Here's how the part is built. I have some questions about the finished solid (model axes, mm). Give positions to 0.01 mm unless a question says otherwise; leave off trailing zeros. Order: outer loops, then holes, each group sorted by start corner. A loop starts at its lowest first (then second) coordinate and runs counter-clockwise, first axis right, second up.
from build123d import *

# Parameters (mm, degrees)
F0_R     = 75
F1_DEPTH = 8


with BuildPart() as f1:
    # F0 (on Top) → F1 (new body)
    with BuildSketch(Plane.XY):
        with BuildLine():
            ThreePointArc((-168.166967, -90.974196), (-117.487432, -76.990459), (-83, -37.309516))
            ThreePointArc((-83, -37.309516), (-48.512568, -76.990459), (2.166967, -90.974196))
            ThreePointArc((2.166967, -90.974196), (84.481738, -33.820644), (64.346717, 64.346717))
            ThreePointArc((64.346717, 64.346717), (-83, 125.379726), (-230.346717, 64.346717))
            ThreePointArc((-230.346717, 64.346717), (-250.481738, -33.820644), (-168.166967, -90.974196))
        make_face()
        with Locations((-166, 0)):
            Circle(F0_R, mode=Mode.SUBTRACT)
        with BuildLine():
            ThreePointArc((-75, 0), (0, 75), (75, 0))
            ThreePointArc((75, 0), (0, -75), (-75, 0))
        make_face(mode=Mode.SUBTRACT)
        with Locations((-166, 0)):
            Circle(F0_R)
        with BuildLine():
            ThreePointArc((2.166967, -90.974196), (-48.512568, -76.990459), (-83, -37.309516))
            ThreePointArc((-83, -37.309516), (-117.487432, -76.990459), (-168.166967, -90.974196))
            Line((-168.166967, -90.974196), (-83.238128, -92.997164))
            ThreePointArc((-83.238128, -92.997164), (-89.98637, -75.845236), (-73, -83))
            ThreePointArc((-73, -83), (-75.845236, -89.98637), (-82.761872, -92.997164))
            Line((-82.761872, -92.997164), (2.166967, -90.974196))
        make_face()
    extrude(amount=F1_DEPTH)


solid = f1.part
Q1. I'm going to push flat-ended pins straight in: P1, Ø1, axis at y = -21.5, z = 2, coming from the -X side; P2, Ø23, axis at x = -83, y = -83, coming from the +Z side; P3, Ø4, axis at y = 25.5, z = 2, coming from the +X side; P4, Ø4, axis at x = 36, z = 2.5, coming from the +Y side. Where does each tip first touch, or does it pass through?
Filled sheet:
P1: stops at x = -254.54
P2: stops at z = 8
P3: stops at x = 87.91
P4: stops at y = 89.43
Q2. I need wall thicknesses on L1, parallel to Y at x = -20.5, z = 2.5; L2, parallel to Y at x = 0, z = 4.5; L3, parallel to X at y = 42.5, z = 0.5. Which ranges of each line are inside material? Lowest first, please.
Filled sheet:
L1: y = -91.51 to -72.14, 72.14 to 115.79
L2: y = -91.03 to -75, 75 to 108.14
L3: x = -246.47 to -61.8, 61.8 to 80.47
Q3. Thinking about a two-plate mould opening in X: for faces 1 (the face through (84, -35, 4)), 2 (the face through (-80.709, 125.367, 3.944)), 3 (the face through (-9.764, -74.362, 3.944)), which applies, released by +X, released by -X, zero draft, split by the parting line, or undercut?
Filled sheet:
face 1: released by +X
face 2: split by the parting line
face 3: undercut
Q4. If we section it at A-A on y = 0: List the corners of the cut face in (x, z) for me, plus the area to 3 significant figures.
Filled sheet:
outline: (-257, 0) - (-75, 0) - (-75, 8) - (-257, 8) - close; (75, 0) - (91, 0) - (91, 8) - (75, 8) - close
area: 1,580 mm2
Q5. If we section it at D-D on x = -161: List the corners of the cut face in (y, z) for me, plus the area to 3 significant figures.
Filled sheet:
outline: (-91.14, 0) - (110.23, 0) - (110.23, 8) - (-91.14, 8) - close
area: 1,610 mm2
Q6. If we section it at B-B on z = 1.75: List the corners of the cut face in (x, y) for me, plus the area to 3 significant figures.
Filled sheet:
outline: (-230.35, 64.35) arc R91 ccw to (-168.17, -90.97) - (-83.24, -93) arc R10 cw (long way) to (-73, -83) arc R10 cw to (-82.76, -93) - (2.17, -90.97) arc R91 ccw to (64.35, 64.35) arc R208.38 ccw to start; hole circle Ø150 at (0, 0)
area: 44,000 mm2
Q7. If we section it at C-C on x = 51.5: List the corners of the cut face in (y, z) for me (3 decimals).
Filled sheet:
outline: (-75.025, 0) - (-54.523, 0) - (-54.523, 8) - (-75.025, 8) - close; (54.523, 0) - (76.16, 0) - (76.16, 8) - (54.523, 8) - close
